Input: dimensioned drawing with shaded views. Units: mm. Origin: part minimum x, y, z. Give positions to 0.01 mm unless a question says otherwise; leave off trailing zeros. Write each loop counter-clockwise with the first axis right and the second up, starting at its lowest first coordinate (ties: lowest second). Pieces come first, ordered by that corner, then holes.
Q1. Line query: line 1 (Y direction, x = 12.7, z = 2); line 2 (X direction, y = 6, z = 1.55); line 3 (X direction, y = 23.5, z = 1.5). Output: solid intervals per line, ascending.
Q2. Section A-A (y = 6.35). Return the cut outline in (x, z) (3 decimals).
Q3. Pin query (flat end, axial travel): pin 1 Ø12 at (x, y) = (60.5, 10.5) entering from -Z. Return the tip coordinate at first contact, or that it passes through.
Q4. Section B-B (x = 76.2). Return the cut outline in (y, z) (3 decimals), plus the area to 3 significant figures.
Q5. Section C-C (z = 2.65). Return the cut outline in (x, y).
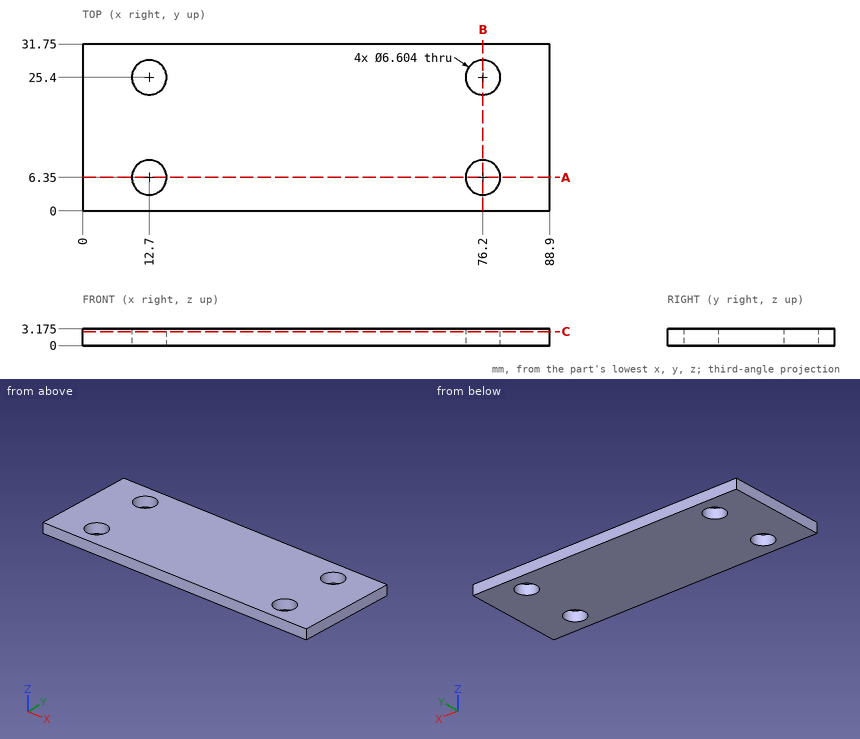
Computed:
1. line 1: y = 0 to 3.05, 9.65 to 22.1, 28.7 to 31.75
1. line 2: x = 0 to 9.42, 15.98 to 72.92, 79.48 to 88.9
1. line 3: x = 0 to 10, 15.4 to 73.5, 78.9 to 88.9
2. outline: (0, 0) - (9.398, 0) - (9.398, 3.175) - (0, 3.175) - close; (16.002, 0) - (72.898, 0) - (72.898, 3.175) - (16.002, 3.175) - close; (79.502, 0) - (88.9, 0) - (88.9, 3.175) - (79.502, 3.175) - close
3. pin 1: stops at z = 0
4. outline: (0, 0) - (3.048, 0) - (3.048, 3.175) - (0, 3.175) - close; (9.652, 0) - (22.098, 0) - (22.098, 3.175) - (9.652, 3.175) - close; (28.702, 0) - (31.75, 0) - (31.75, 3.175) - (28.702, 3.175) - close
4. area: 58.9 mm2
5. outline: (0, 0) - (88.9, 0) - (88.9, 31.75) - (0, 31.75) - close; hole circle Ø6.6 at (12.7, 6.35); hole circle Ø6.6 at (12.7, 25.4); hole circle Ø6.6 at (76.2, 6.35); hole circle Ø6.6 at (76.2, 25.4)
